Could you check a few things on this model? Use its own coordinates, in mm. A direction names the side the tool comes from. Round coordinates to 2 decimals unless told otherwise and drop trailing zeros. Loops run counter-clockwise (first coordinate to the right, second up) from the corner with the lowest first, then second, coordinate; pieces in that order, holes last. Notation, with made-up numbers: (55, -25) - (112, -25) arc R26 cw to (112, 14) - close; hole circle Ø7 at (47.5, 75). An arc over 180 degrees is marked (long way). Put each result on its own line as item: value. Start each with the question number.
from build123d import *

# Parameters (mm, degrees)
EXTRUDE_1_DEPTH      = 1.2
SKETCH_2_R           = 1.375
SKETCH_2_R_2         = 1.15
CUT_EXTRUDE_1_DEPTH  = 2.2
SKETCH_3_W           = 13.1
SKETCH_3_H           = 10
EXTRUDE_2_DEPTH      = 3.2
EXTRUDE_2_DEPTH_BACK = 2.5
SKETCH_4_W           = 5.3
SKETCH_4_H           = 5.3
EXTRUDE_3_DEPTH      = 5.5


with BuildPart() as part:
    # Эскиз1 → Бобышка-Вытянуть1 (new body)
    with BuildSketch(Plane(origin=(0, 0, 0), x_dir=(1, 0, 0), z_dir=(0, 1, 0))):
        Polygon((0, 0), (0, 29), (47, 29), (47, 20), (73.1, 13.5), (73.1, 1.5), (56.2, 1.5), (56.2, 0), align=None)
    extrude(amount=EXTRUDE_1_DEPTH)

    # Эскиз2 → Вырез-Вытянуть1 (cut, through all)
    with BuildSketch(Plane(origin=(0, 1.2, 0), x_dir=(1, 0, 0), z_dir=(0, 1, 0))):
        with Locations((2.675, 16.025)):
            Circle(SKETCH_2_R)
        with Locations((67.725, 7.025)):
            Circle(SKETCH_2_R)
        with Locations((34.75, 6.4)):
            Circle(SKETCH_2_R_2)
    extrude(amount=-CUT_EXTRUDE_1_DEPTH, mode=Mode.SUBTRACT)

    # Эскиз3 → Бобышка-Вытянуть2 (add, two sides)
    with BuildSketch(Plane(origin=(0, 1.2, 0), x_dir=(1, 0, 0), z_dir=(0, 1, 0))) as extrude_2_sk:
        with Locations((16.9, 24.85)):
            Rectangle(SKETCH_3_W, SKETCH_3_H)
        with Locations((36.9, 24.85)):
            Rectangle(SKETCH_3_W, SKETCH_3_H)
    extrude(amount=EXTRUDE_2_DEPTH)
    extrude(extrude_2_sk.sketch, amount=-EXTRUDE_2_DEPTH_BACK)

    # Эскиз4 → Бобышка-Вытянуть3 (add)
    with BuildSketch(Plane.XZ):
        with Locations((18.15, -8.15)):
            Rectangle(SKETCH_4_W, SKETCH_4_H)
    extrude(amount=EXTRUDE_3_DEPTH)


solid = part.part
Item 1: Suppose I cut it at D-D, the plane x = 46. List the corners of the cut face in (y, z) for me.
Item 2: Suppose I cut it at B-B, the plane x = 34.75. List the corners of the cut face in (y, z) for me, then the cut area to 3 significant figures.
Item 3: Thinking about a two-plate mould opening in X: for faces 4 (the face through (59.867, 0.592, -16.796)), 5 (the face through (66.634, 0.608, -6.188)), 6 (the face through (27, 1, -29)), 7 (the face through (17, -1.3, -25)), which applies, released by +X, released by -X, zero draft, split by the parting line, or undercut?
Item 4: I need wall thicknesses on line 1 (Z direction, x = 34.75, y = 0.35); line 2 (Z direction, x = 21, y = 3.25); line 3 (Y direction, x = 28.5, z = -16.25). Which ranges of each line are inside material? Lowest first, please. Write a range as from..to.
Item 5: Suppose I cut it at C-C, the plane z = -11.5. List the corners of the cut face in (x, y) for me.
Item 6: Will these pins go through, and if not, where does the flat tip stop? P1, Ø1, axis at x = 37.5, z = -4, coming from the +Y side; P2, Ø5, axis at y = 0.5, z = -24, coming from the +X side; P3, Ø0.6, axis at x = 7.5, y = 0.5, coming from the -Z side.
Item 7: On a 3-axis mill with a long thin cutter (end or side, diameter ignored), from which of +Z, -Z, +X, -X, +Y, -Y can I reach the whole of each face in a straight line? I mean faces 1 (the face through (45, 1, -29)), 2 (the face through (18, -3, -5.5)), 3 (the face through (65, 1, -1.5)). Say none if no direction works.
Item 8: Suppose I cut it at A-A, the plane y = 2.5. List the corners of the cut face in (x, z) for me.
Numbers:
1. outline: (0, -29) - (1.2, -29) - (1.2, 0) - (0, 0) - close
2. outline: (-1.3, -29.85) - (4.4, -29.85) - (4.4, -19.85) - (1.2, -19.85) - (1.2, -7.55) - (0, -7.55) - (0, -19.85) - (-1.3, -19.85) - close; (0, -5.25) - (1.2, -5.25) - (1.2, 0) - (0, 0) - close
2. area: 78.1 mm^2
3. face 4: released by +X
3. face 5: undercut
3. face 6: undercut
3. face 7: zero draft
4. line 1: -29.85..-7.55, -5.25..0
4. line 2: -29.85..-19.85
4. line 3: 0..1.2
5. outline: (0, 0) - (73.1, 0) - (73.1, 1.2) - (0, 1.2) - close
6. P1: y = 1.2
6. P2: x = 47
6. P3: z = -29
7. face 1: -Z, +X, +Y, -Y
7. face 2: +Z, +X, -X, -Y
7. face 3: +Z, +X, +Y, -Y
8. outline: (10.35, -29.85) - (23.45, -29.85) - (23.45, -19.85) - (10.35, -19.85) - close; (30.35, -29.85) - (43.45, -29.85) - (43.45, -19.85) - (30.35, -19.85) - close
